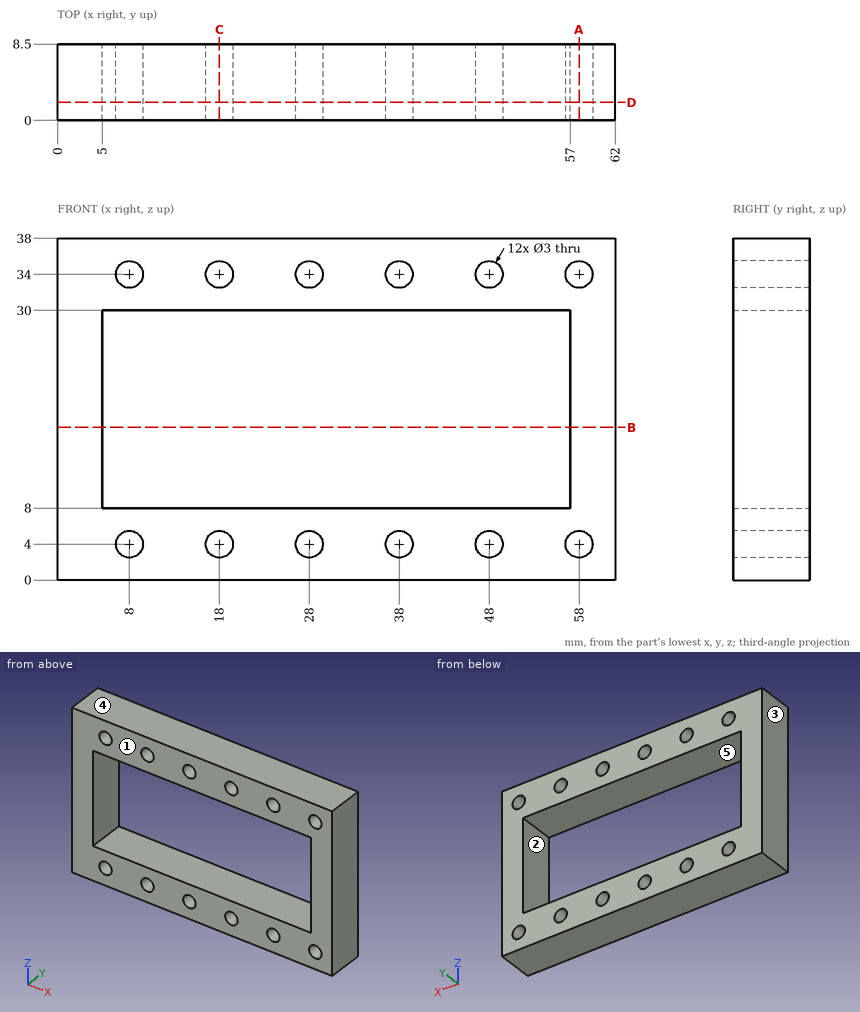
Drawing for the job (mm, zero at the part's lowest x, y, z). A direction names the side the tool comes from. Coordinates: 2 decimals unless noted, no trailing zeros. Order: outer loops, then holes, each group sorted by start corner. A loop starts at its lowest first (then second) coordinate and runs counter-clockwise, first axis right, second up. Notation, with made-up numbers: (55.5, -14) -> (83.5, -14) arc R15 ccw to (83.5, 8) -> close; hole circle Ø7 at (72.5, -38.75). An arc over 180 degrees is marked (long way). Return JSON: item names as keys, results as strings.
Item 1: Mould opens along Z. For the marked faces 3, 4 and 5 say: pulls with the +Z half, pulls with the -Z half, needs draft (parallel to the pull), parting line crosses it, or undercut.
Model answer:
{"face 3": "needs draft", "face 4": "pulls with the +Z half", "face 5": "undercut"}
Item 2: Wall check: line 1 along Z through (x, y) = (58, 6); line 2 along Z through (x, y) = (28, 5.25); line 3 along X through (y, z) = (4, 18). Give the ranges that are in metal, low to high. Write a range as from..to.
Model answer:
{"line 1": "z = 0..2.5, 5.5..32.5, 35.5..38", "line 2": "z = 0..2.5, 5.5..8, 30..32.5, 35.5..38", "line 3": "x = 0..5, 57..62"}
Item 3: Slice it at A-A (x = 58). Write the cut outline in (y, z).
Model answer:
{"outline": "(0, 0) -> (8.5, 0) -> (8.5, 2.5) -> (0, 2.5) -> close; (0, 5.5) -> (8.5, 5.5) -> (8.5, 32.5) -> (0, 32.5) -> close; (0, 35.5) -> (8.5, 35.5) -> (8.5, 38) -> (0, 38) -> close"}
Item 4: 3-axis set-ups, long thin cutter, end or side, ignore diameter. For the marked faces 1 and 2: which of +Z, -Z, +X, -X, +Y, -Y reach the whole face in a straight line?
Model answer:
{"face 1": "+Z, -Z, +X, -X, -Y", "face 2": "+Y, -Y"}
Item 5: Slice it at B-B (z = 17). Write the cut outline in (x, y).
Model answer:
{"outline": "(0, 0) -> (5, 0) -> (5, 8.5) -> (0, 8.5) -> close; (57, 0) -> (62, 0) -> (62, 8.5) -> (57, 8.5) -> close"}
Item 6: Pin check, flat tips, straight feed: P1, Ø4, axis at x = 8, z = 4, coming from the -Y side; P2, Ø1.8, axis at x = 48, z = 4, coming from the +Y side. Stop position of each tip, or through.
Model answer:
{"P1": "stops at y = 0", "P2": "passes through"}
Item 7: Slice it at C-C (x = 18). Write the cut outline in (y, z).
Model answer:
{"outline": "(0, 0) -> (8.5, 0) -> (8.5, 2.5) -> (0, 2.5) -> close; (0, 5.5) -> (8.5, 5.5) -> (8.5, 8) -> (0, 8) -> close; (0, 30) -> (8.5, 30) -> (8.5, 32.5) -> (0, 32.5) -> close; (0, 35.5) -> (8.5, 35.5) -> (8.5, 38) -> (0, 38) -> close"}
Item 8: Slice it at D-D (y = 2). Count the separate pieces of the cut face and the enclosed holes in it, then the cut area to 3 significant figures.
Model answer:
{"separate pieces": "1", "enclosed holes": "13", "area": "1,130 mm²"}
